```python
from build123d import *

# Parameters (mm, degrees)
SKETCH1_R           = 25
BOSS_EXTRUDE1_DEPTH = 3
FILLET1_R           = 5
SKETCH9_R           = 25
BOSS_EXTRUDE2_DEPTH = 3


with BuildPart() as part:
    # Sketch1 → Boss-Extrude1 (new body)
    with BuildSketch(Plane(origin=(0, 0, 0), x_dir=(1, 0, 0), z_dir=(0, 1, 0))):
        with Locations(Location((0, 0, 0), (0, 0, 270))):
            Circle(SKETCH1_R)
    extrude(amount=BOSS_EXTRUDE1_DEPTH)

    # Fillet1
    # the kernel refuses this fillet: 5 mm, written as the material it takes off along each edge
    with BuildSketch(Plane(origin=(0, 3, 0), x_dir=(0, 0, 1), z_dir=(-1, 0, 0))) as fillet1_piece_1:
        with BuildLine():
            CenterArc((20.417424305, -5), FILLET1_R, 23.578178478, 66.421821522)
            Line((20.417424305, 0), (20.417424305, 0.1))
            Line((20.417424305, 0.1), (25, 0.1))
            Line((25, 0.1), (25.1, 0))
            ThreePointArc((25.1, 0), (25.1, -1.5), (25.091651514, -2.96))
            Line((25.091651514, -2.96), (25, -3))
        make_face()
    revolve(axis=Axis((0, 3, 0), (0, 1, 0)), mode=Mode.SUBTRACT)

    # Sketch9 → Boss-Extrude2 (add)
    with BuildSketch(Plane.XZ):
        with Locations(Location((0, 0, 0), (0, 0, 270))):
            Circle(SKETCH9_R)
    extrude(amount=BOSS_EXTRUDE2_DEPTH)


solid = part.part
```
Input: part model. Units: mm. Frame: model coordinates. Round coordinates to 2 decimals unless told otherwise and drop trailing zeros. Loops run counter-clockwise (first coordinate to the right, second up) from the corner with the lowest first, then second, coordinate; pieces in that order, holes last. Notation, with made-up numbers: (-24, -30) - (7, -30) arc R26 ccw to (7, -4) - close; hole circle Ø11 at (89.25, 36). An arc over 180 degrees is marked (long way). One line per item, written item: value. Start each with the question number.
(1) Contact query for a flat-ended pin moving along its axis: P1, Ø3, axis at x = -1, y = 1.5, coming from the -Z side. Output: stop coordinate, or through.
(2) Ray query, line 1 (Y direction, x = -20, z = -5); line 2 (Z direction, x = -0.5, y = -2) (3 decimals); line 3 (Z direction, x = -17, y = -2.55). Return the intervals inside material, ascending. Write a range as [from, to].
(3) Section A-A, the plane y = -0.6. Return loops of the section in (x, z).
(4) Section C-C, the plane z = 0. Return loops of the section in (x, y).
(5) Section B-B, the plane x = 0. Return loops of the section in (y, z).
Results below:
1. P1: z = -24.98
2. line 1: [-3, 3]
2. line 2: [-24.995, 24.995]
2. line 3: [-18.33, 18.33]
3. outline: circle Ø50 at (0, 0)
4. outline: (-25, -3) - (25, -3) - (25, 0) arc R5 ccw to (20.42, 3) - (-20.42, 3) arc R5 ccw to (-25, 0) - close
5. outline: (-3, -25) - (0, -25) arc R5 ccw to (3, -20.42) - (3, 20.42) arc R5 ccw to (0, 25) - (-3, 25) - close
